```python
from build123d import *

# Parameters (mm, degrees)
SKETCH1_R           = 2.75
SKETCH1_R_2         = 1.75
BOSS_EXTRUDE1_DEPTH = 5
CUT_EXTRUDE1_DEPTH  = 2.5


with BuildPart() as part:
    # Sketch1 → Boss-Extrude1 (new body)
    with BuildSketch(Plane.XY):
        with BuildLine():
            Line((445.881443411, -1323.745162979), (445.881443411, -1203.505162979))
            ThreePointArc((445.881443411, -1203.505162979), (444.891464332, -1201.115142059), (442.501443411, -1200.125162979))
            Line((442.501443411, -1200.125162979), (361.261443411, -1200.125162979))
            ThreePointArc((361.261443411, -1200.125162979), (358.871422491, -1201.115142059), (357.881443411, -1203.505162979))
            Line((357.881443411, -1203.505162979), (357.881443411, -1323.745162979))
            ThreePointArc((357.881443411, -1323.745162979), (358.871422491, -1326.1351839), (361.261443411, -1327.125162979))
            Line((361.261443411, -1327.125162979), (442.501443411, -1327.125162979))
            ThreePointArc((442.501443411, -1327.125162979), (444.891464332, -1326.1351839), (445.881443411, -1323.745162979))
        make_face()
        with Locations((371.881443411, -1233.625162979)):
            Circle(SKETCH1_R, mode=Mode.SUBTRACT)
        with Locations((431.881443411, -1233.625162979)):
            Circle(SKETCH1_R, mode=Mode.SUBTRACT)
        with Locations((371.881443411, -1293.625162979)):
            Circle(SKETCH1_R, mode=Mode.SUBTRACT)
        with Locations((431.881443411, -1293.625162979)):
            Circle(SKETCH1_R, mode=Mode.SUBTRACT)
        with Locations((386.881443411, -1203.515162979)):
            Circle(SKETCH1_R_2, mode=Mode.SUBTRACT)
        with Locations((416.881443411, -1203.515162979)):
            Circle(SKETCH1_R_2, mode=Mode.SUBTRACT)
    extrude(amount=BOSS_EXTRUDE1_DEPTH)

    # Sketch2 → Cut-Extrude1 (cut)
    with BuildSketch(Plane.XY.offset(5)):
        Polygon((388.469156651, -1200.765162979), (385.293730171, -1200.765162979), (383.706016931, -1203.515162979), (385.293730171, -1206.265162979), (388.469156651, -1206.265162979), (390.056869892, -1203.515162979), align=None)
        Polygon((418.469156651, -1200.765162979), (415.293730171, -1200.765162979), (413.706016931, -1203.515162979), (415.293730171, -1206.265162979), (418.469156651, -1206.265162979), (420.056869892, -1203.515162979), align=None)
    extrude(amount=-CUT_EXTRUDE1_DEPTH, mode=Mode.SUBTRACT)


solid = part.part
```
CAD build for the part. Positions are in the model's coordinates, mm. A direction names the side the tool comes from. Give positions to 0.01 mm unless a question says otherwise; leave off trailing zeros.
(1) Mould opens along Y. For faces 1 (the flat face through (402, -1200.125, 2)), 2 (the cylindrical face through (415.493, -1204.58, 1.232)), 3 (the cylindrical face through (358.845, -1326.109, 2.465)), 4 (the flat face through (414.51, -1202.12, 3.77)) say: released by +Y, released by -Y, zero draft, split by the parting line, or undercut.
(2) Flat gauge pin, fed straight in: pin 1 (3 mm diameter, centred on x = 386.88, y = -1203.52, fed in from -Z). Where does the tip first touch, or does it go through?
(3) Tool access for faces 5 (the cylindrical face through (431.29, -1236.31, 2.46)), 6 (the flat face through (384.49, -1204.87, 3.77)): list every direction of +Z, -Z, +X, -X, +Y, -Y with a clear straight run to the whole face (end or side of a thin tool).
(4) Drill centre lines: L1, parallel to X at y = -1234.5, z = 3.45; L2, parallel to X at y = -1231.5, z = 1.4; L3, parallel to Y at x = 385, z = 2.85. Where is each one in solid material? Low to high.
Results found:
1. face 1: released by +Y
1. face 2: undercut
1. face 3: released by -Y
1. face 4: undercut
2. pin 1: passes through
3. face 5: +Z, -Z
3. face 6: +Z
4. L1: x = 357.88 to 369.27, 374.49 to 429.27, 434.49 to 445.88
4. L2: x = 357.88 to 370.14, 373.63 to 430.14, 433.63 to 445.88
4. L3: y = -1327.13 to -1205.76, -1201.27 to -1200.13
